Part print with two shaded views. Sizes in mm from the minimum x, y, z corner. A direction names the side the tool comes from. Round coordinates to 2 decimals unless told otherwise and drop trailing zeros. Write each loop counter-clockwise with the first axis right and the second up, starting at its lowest first coordinate (ties: lowest second). Pieces come first, ordered by that corner, then holes. Notation, with made-up numbers: (73, 23.5) -> (132, 23.5) arc R29 ccw to (132, 58.5) -> close; hole circle Ø4 at (82, -5.5). An arc over 180 degrees is marked (long way). Return JSON: item names as keys, results as strings. Group by question number.
(1) Tool access for the marked faces 1, 2 and 3: list every direction of +Z, -Z, +X, -X, +Y, -Y with a clear straight run to the whole face (end or side of a thin tool).
(2) Saw through at B-B (y = 10). List the corners of the cut face in (x, z).
(3) Drill centre lines: L1, parallel to Y at x = 2.5, z = 34.05; L2, parallel to X at y = 5, z = 34.2; L3, parallel to Z at x = 8, y = 14.5. Where is each one in solid material? Low to high. Write a range as from..to.
(4) Drop flat-ended pins along their axis: pin 1 Ø6.5 at (y, z) = (9.5, 39) entering from -X; pin 2 Ø7 at (x, y) = (2.5, 15) entering from -Z; pin 3 Ø3.5 at (x, y) = (50, 12) entering from +Z. Give the stop position or say it passes through.
(5) Saw through at D-D (z = 40). List the corners of the cut face in (x, y), plus the area to 3 significant figures.
(6) Saw through at C-C (x = 37.25). List the corners of the cut face in (y, z), plus the area to 4 significant figures.
(7) Saw through at A-A (x = 52). List the corners of the cut face in (y, z).
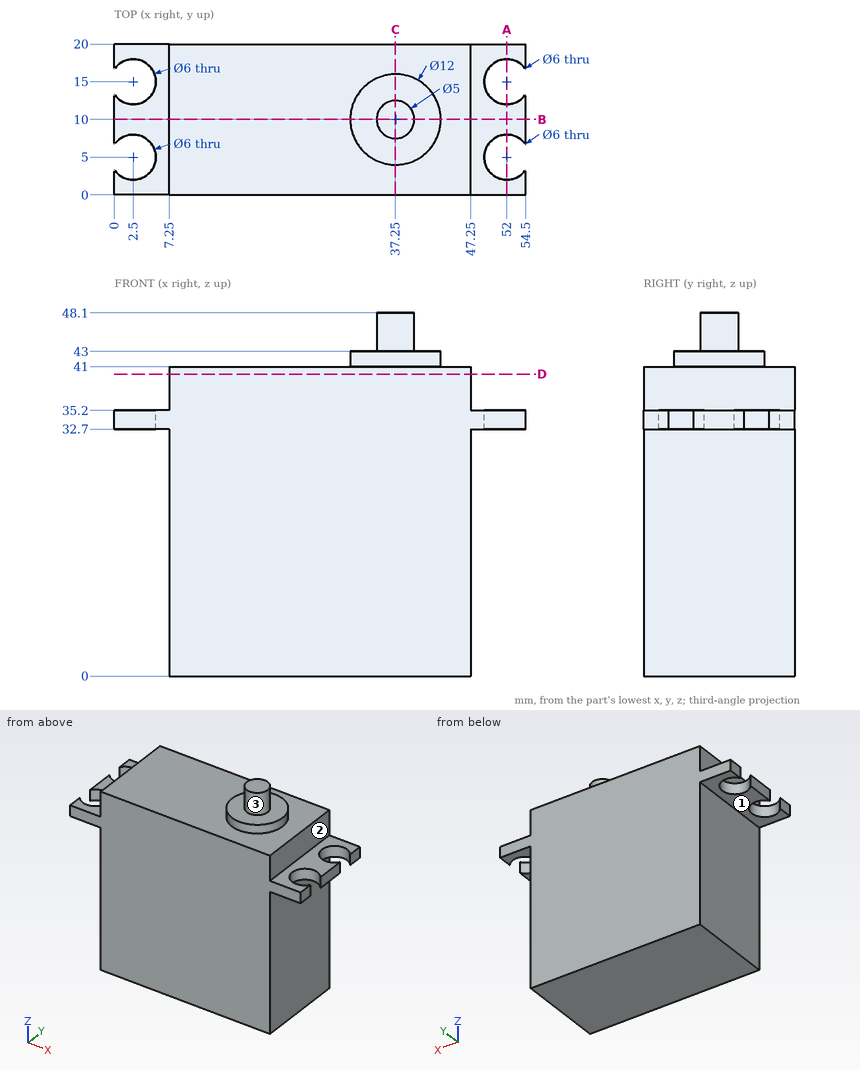
Computed values:
{
 "1": {"face 1": "-Z, -X, +Y, -Y", "face 2": "+Z, +X, +Y, -Y", "face 3": "+Z"},
 "2": {"outline": "(0, 32.7) -> (7.25, 32.7) -> (7.25, 0) -> (47.25, 0) -> (47.25, 32.7) -> (54.5, 32.7) -> (54.5, 35.2) -> (47.25, 35.2) -> (47.25, 41) -> (43.25, 41) -> (43.25, 43) -> (39.75, 43) -> (39.75, 48.1) -> (34.75, 48.1) -> (34.75, 43) -> (31.25, 43) -> (31.25, 41) -> (7.25, 41) -> (7.25, 35.2) -> (0, 35.2) -> close"},
 "3": {"L1": "0..2, 8..12, 18..20", "L2": "5.5..49", "L3": "0..41"},
 "4": {"pin 1": "x = 7.25", "pin 2": "z = 32.7", "pin 3": "z = 35.2"},
 "5": {"outline": "(7.25, 0) -> (47.25, 0) -> (47.25, 20) -> (7.25, 20) -> close", "area": "800 mm2"},
 "6": {"outline": "(0, 0) -> (20, 0) -> (20, 41) -> (16, 41) -> (16, 43) -> (12.5, 43) -> (12.5, 48.1) -> (7.5, 48.1) -> (7.5, 43) -> (4, 43) -> (4, 41) -> (0, 41) -> close", "area": "869.5 mm2"},
 "7": {"outline": "(0, 32.7) -> (2, 32.7) -> (2, 35.2) -> (0, 35.2) -> close; (8, 32.7) -> (12, 32.7) -> (12, 35.2) -> (8, 35.2) -> close; (18, 32.7) -> (20, 32.7) -> (20, 35.2) -> (18, 35.2) -> close"}
}
